Geometry check sheet. Reference: the model listing, model coordinates, mm. A direction names the side the tool comes from. Coordinates: 2 decimals unless noted, no trailing zeros.
from build123d import *

# Parameters (mm, degrees)
F1_DEPTH = 11.1125
F2_R     = 6.35


# Not quite as in the source:
# - a feature names something its author has since deleted; it is built from what else it names


with BuildPart() as f1:
    # F0 (on Top) → F1 (new body)
    with BuildSketch(Plane.XY):
        Polygon((-263.525, -101.6), (-263.525, -127), (80.9498, -127), (92.075, -127), (263.525, -127), (263.525, -101.6), (263.525, 127), (92.075, 127), (92.075, 101.6), (80.9498, 101.6), (80.9498, 127), (-80.9498, 127), (-80.9498, 101.6), (-92.075, 101.6), (-92.075, 127), (-263.525, 127), align=None)
    extrude(amount=F1_DEPTH)

    # F2
    f2_edges = [f1.edges().sort_by_distance(p)[0] for p in [
        (263.525, -127, 5.55625),
        (263.525, 127, 5.55625),
        (-263.525, -127, 5.55625),
        (-263.525, 127, 5.55625),
    ]]
    fillet(f2_edges, radius=F2_R)


solid = f1.part
(1) Gauge pin test, flat end, axial feed: pin 1 Ø5.5 at (x, z) = (87, 4) entering from +Y. Record the tip position at first contact, or that the pin passes through.
Findings:
pin 1: stops at y = 101.6
(2) Access from +Z, -Z, +X, -X, +Y, -Y to the whole of each face (thin tool, end or side, straight path). Record for faces 1 (the flat face through (80.95, 114, 5)), 2 (the flat face through (-4, -127, 5)).
Findings:
face 1: +Z, -Z, +Y
face 2: +Z, -Z, +X, -X, -Y
(3) Scan line: L1, parallel to X at y = 114.5, z = 3.5 (3 decimals). Record every from-to range of solid material in increasing order.
Findings:
L1: x = -263.525 to -92.075, -80.95 to 80.95, 92.075 to 263.525
(4) Draft check along X on faces 3 (the flat face through (-92.075, 114, 5)), 4 (the flat face through (1, 127, 5)), 5 (the flat face through (92.075, 114, 5)), 6 (the flat face through (263.525, -2, 5)). Enter one of: +X half, -X half, draft (parallel to the pull), parting line (faces both ways), or undercut.
Findings:
face 3: undercut
face 4: draft
face 5: undercut
face 6: +X half
